```python
from build123d import *

# Parameters (mm, degrees)
SKETCH1_W                      = 90
SKETCH1_H                      = 20
BASE_FLANGE1_DEPTH             = 3
EDGE_FLANGE1_STRIP_W           = 17.2
EDGE_FLANGE1_STRIP_H           = 3
EDGE_FLANGE1_STRIP_CUT_DEPTH   = 20
EDGE_FLANGE1_STRIP_2_W         = 17.2
EDGE_FLANGE1_STRIP_2_H         = 3
EDGE_FLANGE1_STRIP_CUT_2_DEPTH = 20
EDGE_FLANGE1_DEPTH             = 20
EDGE_FLANGE1_BEND_DEPTH        = 20
CUT_EXTRUDE1_DEPTH             = 10
CUT_EXTRUDE2_START             = -10
CUT_EXTRUDE2_DEPTH             = 10


# Sheet-metal steps are written as plain solids
with BuildPart() as part:
    # Sketch1 → Base-Flange1 (new body)
    with BuildSketch(Plane.XY):
        Rectangle(SKETCH1_W, SKETCH1_H)
    extrude(amount=-BASE_FLANGE1_DEPTH)

    # Edge-Flange1 strip (across the edge) → Edge-Flange1 strip cut (cut)
    with BuildSketch(Plane(origin=(45, -10, 0), x_dir=(-1, 0, 0), z_dir=(0, 1, 0))):
        with Locations((-3, -1.5)):
            Rectangle(EDGE_FLANGE1_STRIP_W, EDGE_FLANGE1_STRIP_H)
    extrude(amount=EDGE_FLANGE1_STRIP_CUT_DEPTH, mode=Mode.SUBTRACT)

    # Edge-Flange1 strip 2 (across the edge) → Edge-Flange1 strip cut 2 (cut)
    with BuildSketch(Plane(origin=(-45, 10, 0), x_dir=(1, 0, 0), z_dir=(0, -1, 0))):
        with Locations((-3, -1.5)):
            Rectangle(EDGE_FLANGE1_STRIP_2_W, EDGE_FLANGE1_STRIP_2_H)
    extrude(amount=EDGE_FLANGE1_STRIP_CUT_2_DEPTH, mode=Mode.SUBTRACT)

    # Edge-Flange1 section (across the edge) → Edge-Flange1 (add)
    with BuildSketch(Plane(origin=(45, -10, 0), x_dir=(-1, 0, 0), z_dir=(0, 1, 0))):
        with BuildLine():
            Line((0, 2.6), (0, 17))
            Line((0, 17), (3, 17))
            Line((3, 17), (3, 2.6))
            ThreePointArc((3, 2.6), (3.761522369, 0.761522369), (5.6, 0))
            Line((5.6, 0), (5.6, -3))
            ThreePointArc((5.6, -3), (1.640202025, -1.359797975), (0, 2.6))
        make_face()
    extrude(amount=EDGE_FLANGE1_DEPTH)

    # Edge-Flange1 section 2 (across the edge) → Edge-Flange1 bend (add)
    with BuildSketch(Plane(origin=(-45, 10, 0), x_dir=(1, 0, 0), z_dir=(0, -1, 0))):
        with BuildLine():
            Line((0, 2.6), (0, 17))
            Line((0, 17), (3, 17))
            Line((3, 17), (3, 2.6))
            ThreePointArc((3, 2.6), (3.761522369, 0.761522369), (5.6, 0))
            Line((5.6, 0), (5.6, -3))
            ThreePointArc((5.6, -3), (1.640202025, -1.359797975), (0, 2.6))
        make_face()
    extrude(amount=EDGE_FLANGE1_BEND_DEPTH)

    # Sketch12 → Cut-Extrude1 (cut)
    with BuildSketch(Plane.ZY.offset(45)):
        with BuildLine():
            Line((11.5, 5), (11.5, -5))
            ThreePointArc((11.5, -5), (10, -6.5), (8.5, -5))
            Line((8.5, -5), (8.5, 5))
            ThreePointArc((8.5, 5), (10, 6.5), (11.5, 5))
        make_face()
    extrude(amount=-CUT_EXTRUDE1_DEPTH, mode=Mode.SUBTRACT)

    # Sketch13 → Cut-Extrude2 (cut)
    with BuildSketch(Plane(origin=(45, 0, 0), x_dir=(0, 0, -1), z_dir=(1, 0, 0)).offset(CUT_EXTRUDE2_START)):
        with BuildLine():
            Line((-8.5, 5), (-8.5, -5))
            ThreePointArc((-8.5, -5), (-10, -6.5), (-11.5, -5))
            Line((-11.5, -5), (-11.5, 5))
            ThreePointArc((-11.5, 5), (-10, 6.5), (-8.5, 5))
        make_face()
    extrude(amount=CUT_EXTRUDE2_DEPTH, mode=Mode.SUBTRACT)


solid = part.part
```
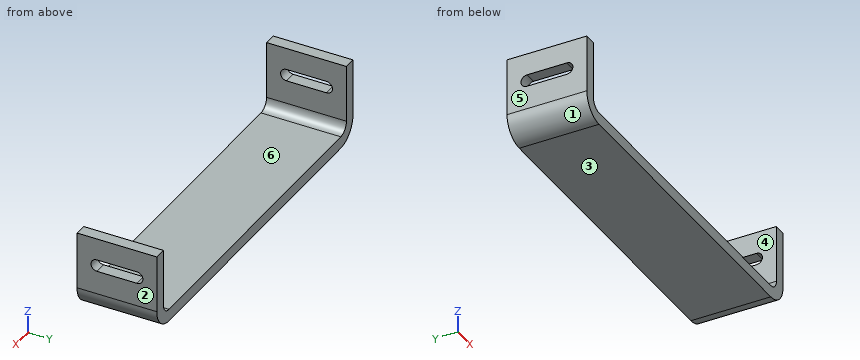
Can you work these out from the model? Positions are in its coordinate system, mm. Face numbers are marked on the shaded views. A direction names the side the tool comes from. Give positions to 0.01 mm unless a question says otherwise; leave off trailing zeros. Order: outer loops, then holes, each group sorted by start corner. A loop starts at its lowest first (then second) coordinate and runs counter-clockwise, first axis right, second up. Notation, with made-up numbers: M 42.25,57.25 L 74.25,57.25 A20 cw 74.25,77.25 Z; hole C 16.5,-38 d6. An arc over 180 degrees is marked long. One line per item, written item: value.
1) Please list where these lines run through material, in increasing order: line 1 along X through (y, z) = (5, 13.5); line 2 along Z through (x, y) = (19.5, -5.75); line 3 along X through (y, z) = (8.25, 0.5).
Answer sheet:
line 1: x = -45 to -42, 42 to 45
line 2: z = -3 to 0
line 3: x = -44.59 to -40.93, 40.93 to 44.59
2) For P1, Ø2, axis at y = 5.5, z = 0.5, coming from the -X side; P2, Ø2, axis at y = 2, z = 1, coming from the +X side; P3, Ø1, axis at x = -30.5, y = 5.5, coming from the +Z side, each with a flat end and sliding along its axis, tell me the tip position at first contact or that it passes through.
Answer sheet:
P1: stops at x = -44.89
P2: stops at x = 44.97
P3: stops at z = 0
3) I want a section at C-C, the plane z = 10. List the corners of the cut face in (x, y) for me, plus the area to 3 significant figures.
Answer sheet:
outline: M -45,-10 L -42,-10 L -42,-6.5 L -45,-6.5 Z; M -45,6.5 L -42,6.5 L -42,10 L -45,10 Z; M 42,-10 L 45,-10 L 45,-6.5 L 42,-6.5 Z; M 42,6.5 L 45,6.5 L 45,10 L 42,10 Z
area: 42.0 mm^2
4) We'd pull the mould along X, two halves only. Please class the marked faces 1, 2, 3 and 4: released by +X, released by -X, zero draft, split by the parting line, or undercut.
Answer sheet:
face 1: released by -X
face 2: released by +X
face 3: zero draft
face 4: undercut
5) I want a section at B-B, the plane y = -3.5. List the corners of the cut face in (x, z) for me.
Answer sheet:
outline: M -45,2.6 A5.6 ccw -39.4,-3 L 39.4,-3 A5.6 ccw 45,2.6 L 45,8.5 L 42,8.5 L 42,2.6 A2.6 cw 39.4,0 L -39.4,0 A2.6 cw -42,2.6 L -42,8.5 L -45,8.5 Z; M -45,11.5 L -42,11.5 L -42,17 L -45,17 Z; M 42,11.5 L 45,11.5 L 45,17 L 42,17 Z
6) I want a section at D-D, the plane y = -8.5. List the corners of the cut face in (x, z) for me.
Answer sheet:
outline: M -45,2.6 A5.6 ccw -39.4,-3 L 39.4,-3 A5.6 ccw 45,2.6 L 45,17 L 42,17 L 42,2.6 A2.6 cw 39.4,0 L -39.4,0 A2.6 cw -42,2.6 L -42,17 L -45,17 Z
7) I want a section at A-A, the plane z = 13.75. List the corners of the cut face in (x, y) for me, plus the area to 3 significant figures.
Answer sheet:
outline: M -45,-10 L -42,-10 L -42,10 L -45,10 Z; M 42,-10 L 45,-10 L 45,10 L 42,10 Z
area: 120 mm^2
8) On a 3-axis mill with a long thin cutter (end or side, diameter ignored), from which of +Z, -Z, +X, -X, +Y, -Y can I reach the whole of each face in a straight line? I mean the marked faces 5 and 6. Say none if no direction works.
Answer sheet:
face 5: +Z, -Z, -X, +Y, -Y
face 6: +Z, +Y, -Y
